```python
from build123d import *

# Parameters (mm, degrees)
SALIENTE_EXTRUIR1_DEPTH = 4
CROQUIS2_W              = 10
CROQUIS2_H              = 4
SALIENTE_EXTRUIR2_DEPTH = 10
CROQUIS3_R              = 1.5
CORTAR_EXTRUIR1_DEPTH   = 10
CROQUIS3_3_R            = 1.5
CORTAR_EXTRUIR2_DEPTH   = 1.65
REDONDEO2_R             = 10
CORTAR_EXTRUIR4_REACH   = 121.7
CROQUIS4_W              = 14.4
CROQUIS4_H              = 16.36262465
CROQUIS4_W_2            = 16.3
CROQUIS4_H_2            = 13.9
CROQUIS4_W_3            = 15.3
CROQUIS4_H_3            = 16.22
CROQUIS5_W              = 56.6
CROQUIS5_H              = 21.54262465
CORTAR_EXTRUIR5_DEPTH   = 4
REDONDEO3_R             = 3
CROQUIS6_W              = 61.43
CROQUIS6_H              = 15.43
CORTAR_EXTRUIR6_DEPTH   = 4
REDONDEO4_R             = 2.22
CROQUIS8_W              = 4
CROQUIS8_H              = 72
CORTAR_EXTRUIR7_DEPTH   = 4


with BuildPart() as part:
    # Croquis1 → Saliente-Extruir1 (new body)
    with BuildSketch(Plane.XY):
        with BuildLine():
            Line((-98, 60), (-98, -4))
            Line((-98, -4), (90, -4))
            Line((90, -4), (90, 60))
            ThreePointArc((90, 60), (88.94427191, 64.472135955), (86, 68))
            Line((86, 68), (-94, 68))
            ThreePointArc((-94, 68), (-96.94427191, 64.472135955), (-98, 60))
        make_face()
    extrude(amount=SALIENTE_EXTRUIR1_DEPTH)

    # Croquis2 → Saliente-Extruir2 (add)
    with BuildSketch(Plane(origin=(0, 0, 0), x_dir=(-1, 0, 0), z_dir=(0, 0, -1))):
        with Locations((46.991549296, 2)):
            Rectangle(CROQUIS2_W, CROQUIS2_H)
        with Locations((-38.991549296, 2)):
            Rectangle(CROQUIS2_W, CROQUIS2_H)
    extrude(amount=SALIENTE_EXTRUIR2_DEPTH)

    # Croquis3 → Cortar-Extruir1 (cut)
    with BuildSketch(Plane.XZ):
        with Locations((38.991549296, -5)):
            Circle(CROQUIS3_R)
        with Locations((-46.991549296, -5)):
            Circle(CROQUIS3_R)
    extrude(amount=-CORTAR_EXTRUIR1_DEPTH, mode=Mode.SUBTRACT)

    # Croquis3<3> → Cortar-Extruir2 (cut)
    # profile 1 of 2: a face of its own
    with BuildSketch(Plane.XZ):
        Polygon((-46.991549296, -8.175426481), (-44.241549296, -6.58771324), (-44.241549296, -3.41228676), (-46.991549296, -1.824573519), (-49.741549296, -3.41228676), (-49.741549296, -6.58771324), align=None)
        with Locations((-46.991549296, -5)):
            Circle(CROQUIS3_3_R, mode=Mode.SUBTRACT)
    # profile 2 of 2: a face of its own
    with BuildSketch(Plane.XZ):
        Polygon((38.991549296, -8.175426481), (41.741549296, -6.58771324), (41.741549296, -3.41228676), (38.991549296, -1.824573519), (36.241549296, -3.41228676), (36.241549296, -6.58771324), align=None)
        with Locations((38.991549296, -5)):
            Circle(CROQUIS3_3_R, mode=Mode.SUBTRACT)
    extrude(amount=-CORTAR_EXTRUIR2_DEPTH, mode=Mode.SUBTRACT)

    # Redondeo2
    # the kernel refuses this fillet: 10 mm, written as the material it takes off along each edge
    with BuildSketch(Plane(origin=(106, 68, 4), x_dir=(0, -1, 0), z_dir=(-1, 0, 0))) as redondeo2_piece_1:
        with BuildLine():
            CenterArc((8, -10), REDONDEO2_R, 90, 53.130102354)
            Line((0, -4), (-0.16, -3.88))
            ThreePointArc((-0.16, -3.88), (-0.2, -2), (-0.2, 0))
            Line((-0.2, 0), (0, 0.2))
            Line((0, 0.2), (8, 0.2))
            Line((8, 0.2), (8, 0))
        make_face()
    extrude(amount=220, mode=Mode.SUBTRACT)

    # Croquis4 → Cortar-Extruir4 (cut, up to next)
    with BuildSketch(Plane(origin=(0, 0, 0), x_dir=(-1, 0, 0), z_dir=(0, 0, -1)), mode=Mode.PRIVATE) as cortar_extruir4_sk1:
        with Locations((-46.4, 18.238687675)):
            Rectangle(CROQUIS4_W, CROQUIS4_H)
    cortar_extruir4_tool1 = extrude(cortar_extruir4_sk1.sketch, amount=-CORTAR_EXTRUIR4_REACH, mode=Mode.PRIVATE) & part.part
    # Croquis4 → Cortar-Extruir4 (cut, up to next)
    with BuildSketch(Plane(origin=(0, 0, 0), x_dir=(-1, 0, 0), z_dir=(0, 0, -1)), mode=Mode.PRIVATE) as cortar_extruir4_sk2:
        with Locations((-65.3, 20.65)):
            Rectangle(CROQUIS4_W_2, CROQUIS4_H_2)
    cortar_extruir4_tool2 = extrude(cortar_extruir4_sk2.sketch, amount=-CORTAR_EXTRUIR4_REACH, mode=Mode.PRIVATE) & part.part
    # Croquis4 → Cortar-Extruir4 (cut, up to next)
    with BuildSketch(Plane(origin=(0, 0, 0), x_dir=(-1, 0, 0), z_dir=(0, 0, -1)), mode=Mode.PRIVATE) as cortar_extruir4_sk3:
        with Locations((-28.5, 19.49)):
            Rectangle(CROQUIS4_W_3, CROQUIS4_H_3)
    cortar_extruir4_tool3 = extrude(cortar_extruir4_sk3.sketch, amount=-CORTAR_EXTRUIR4_REACH, mode=Mode.PRIVATE) & part.part
    add(cortar_extruir4_tool1.solids().sort_by_distance((46.4, 18.238688, 0))[0], mode=Mode.SUBTRACT)
    add(cortar_extruir4_tool2.solids().sort_by_distance((65.3, 20.65, 0))[0], mode=Mode.SUBTRACT)
    add(cortar_extruir4_tool3.solids().sort_by_distance((28.5, 19.49, 0))[0], mode=Mode.SUBTRACT)

    # Croquis5 → Cortar-Extruir5 (cut)
    with BuildSketch(Plane.XY.offset(4)):
        with Locations((47.15, 18.828687675)):
            Rectangle(CROQUIS5_W, CROQUIS5_H)
    extrude(amount=-CORTAR_EXTRUIR5_DEPTH, mode=Mode.SUBTRACT)

    # Redondeo3
    redondeo3_edges = [part.edges().sort_by_distance(p)[0] for p in [
        (75.45, 29.6, 2),
        (75.45, 8.05737535, 2),
        (18.85, 8.05737535, 2),
        (18.85, 29.6, 2),
    ]]
    fillet(redondeo3_edges, radius=REDONDEO3_R)

    # Croquis6 → Cortar-Extruir6 (cut)
    with BuildSketch(Plane.XY.offset(4)):
        with Locations((-43.885, 51.885)):
            Rectangle(CROQUIS6_W, CROQUIS6_H)
    extrude(amount=-CORTAR_EXTRUIR6_DEPTH, mode=Mode.SUBTRACT)

    # Redondeo4
    redondeo4_edges = [part.edges().sort_by_distance(p)[0] for p in [
        (-13.17, 59.6, 2),
        (-13.17, 44.17, 2),
        (-74.6, 44.17, 2),
        (-74.6, 59.6, 2),
    ]]
    fillet(redondeo4_edges, radius=REDONDEO4_R)

    # Croquis8 → Cortar-Extruir7 (cut)
    with BuildSketch(Plane.XY.offset(4)):
        with Locations((88, 32)):
            Rectangle(CROQUIS8_W, CROQUIS8_H)
        with Locations((-96, 32)):
            Rectangle(CROQUIS8_W, CROQUIS8_H)
    extrude(amount=-CORTAR_EXTRUIR7_DEPTH, mode=Mode.SUBTRACT)


solid = part.part
```
Build history of the part. All positions in model axes, mm. A direction names the side the tool comes from. Give positions to 0.01 mm unless a question says otherwise; leave off trailing zeros. Loops run counter-clockwise (first coordinate to the right, second up) from the corner with the lowest first, then second, coordinate; pieces in that order, holes last.
Item 1: Slice it at A-A, the plane x = 51.5. List the corners of the cut face in (y, z), and give its area (3 significant figures).
Answers follow:
outline: (-4, 0) - (8.06, 0) - (8.06, 4) - (-4, 4) - close; (29.6, 0) - (68, 0) arc R10 ccw to (60, 4) - (29.6, 4) - close
area: 192 mm2
Item 2: Slice it at D-D, the plane x = 10. List the corners of the cut face in (y, z), and give its area (3 significant figures).
Answers follow:
outline: (-4, 0) - (68, 0) arc R10 ccw to (60, 4) - (-4, 4) - close
area: 278 mm2
Item 3: Drill centre lines: line 1 (X direction, y = 15.5, z = 1); line 2 (Z direction, x = -30, y = 20); line 3 (Y direction, x = 41, z = -3.25). Where is each one in solid material? Low to high.
Answers follow:
line 1: x = -94 to 18.85, 75.45 to 86
line 2: z = 0 to 4
line 3: y = 1.65 to 4
Item 4: Slice it at B-B, the plane y = 52. List the corners of the cut face in (x, z).
Answers follow:
outline: (-94, 0) - (-74.6, 0) - (-74.6, 4) - (-94, 4) - close; (-13.17, 0) - (86, 0) - (86, 4) - (-13.17, 4) - close
Item 5: Slice it at C-C, the plane y = 33.5. List the corners of the cut face in (x, z).
Answers follow:
outline: (-94, 0) - (86, 0) - (86, 4) - (-94, 4) - close
Item 6: Flat gauge pins, fed straight in: pin 1 (2 mm diameter, centred on x = -36.5, z = 2.5, fed in from +Y); pin 2 (3 mm diameter, centred on y = 1.5, z = -5.5, fed in from +X); pin 3 (4.5 mm diameter, centred on y = 1.5, z = -4.5, fed in from -X). Where does each tip first touch, or does it go through?
Answers follow:
pin 1: stops at y = 66.61
pin 2: stops at x = 43.99
pin 3: stops at x = -51.99
Item 7: Pull direction X, two halves, no side cores. Call faces 5 (the face through (-13.17, 52, 2)), 6 (the face through (-47, 2, -10)), 7 (the face through (43.992, 2, -5)): released by +X, released by -X, zero draft, split by the parting line, or undercut.
Answers follow:
face 5: undercut
face 6: zero draft
face 7: released by +X
Item 8: Which spindle directions (+Z, -Z, +X, -X, +Y, -Y) get a long thin tool onto all of the face, cutting with end or side? Do faces 1 (the face through (19.75, 28.74, 1.97)), 2 (the face through (33.992, 2, -5)), 3 (the face through (-51.992, 2, -5)), 4 (the face through (-44.7, 0, -2.7)). Say none if no direction does.
Answers follow:
face 1: +Z, -Z
face 2: -Z, +Y, -Y
face 3: -Z, -X, +Y, -Y
face 4: -Z, +X, -X, -Y
